from build123d import *

# Parameters (mm, degrees)
CROQUIS1_R              = 12.5
CROQUIS1_R_2            = 0.75
SALIENTE_EXTRUIR1_DEPTH = 10
CROQUIS2_R              = 7.875
SALIENTE_EXTRUIR2_DEPTH = 13
SALIENTE_EXTRUIR3_DEPTH = 8
CROQUIS4_R              = 2
CORTAR_EXTRUIR1_DEPTH   = 32
REDONDEO1_R             = 1


with BuildPart() as part:
    # Croquis1 → Saliente-Extruir1 (new body)
    with BuildSketch(Plane(origin=(0, 0, 0), x_dir=(1, 0, 0), z_dir=(0, 1, 0))):
        Circle(CROQUIS1_R)
        with Locations((7, 0)):
            Circle(CROQUIS1_R_2, mode=Mode.SUBTRACT)
        with Locations((0, -7)):
            Circle(CROQUIS1_R_2, mode=Mode.SUBTRACT)
        with Locations((-7, 0)):
            Circle(CROQUIS1_R_2, mode=Mode.SUBTRACT)
        with Locations((0, 7)):
            Circle(CROQUIS1_R_2, mode=Mode.SUBTRACT)
    extrude(amount=SALIENTE_EXTRUIR1_DEPTH)

    # Croquis2 → Saliente-Extruir2 (add)
    with BuildSketch(Plane(origin=(0, 10, 0), x_dir=(1, 0, 0), z_dir=(0, 1, 0))):
        Circle(CROQUIS2_R)
    extrude(amount=SALIENTE_EXTRUIR2_DEPTH)

    # Croquis3 → Saliente-Extruir3 (add)
    with BuildSketch(Plane(origin=(0, 23, 0), x_dir=(1, 0, 0), z_dir=(0, 1, 0))):
        Polygon((7.5, 0), (3.75, 6.495190528), (-3.75, 6.495190528), (-7.5, 0), (-3.75, -6.495190528), (3.75, -6.495190528), align=None)
    extrude(amount=SALIENTE_EXTRUIR3_DEPTH)

    # Croquis4 → Cortar-Extruir1 (cut, through all)
    with BuildSketch(Plane(origin=(0, 31, 0), x_dir=(1, 0, 0), z_dir=(0, 1, 0))):
        Circle(CROQUIS4_R)
    extrude(amount=-CORTAR_EXTRUIR1_DEPTH, mode=Mode.SUBTRACT)

    # Redondeo1
    redondeo1_edges = [part.edges().sort_by_distance(p)[0] for p in [
        (5.625, 31, 3.247595264),
        (5.625, 31, -3.247595264),
        (0, 31, -6.495190528),
        (-5.625, 31, -3.247595264),
        (-5.625, 31, 3.247595264),
        (0, 31, 6.495190528),
        (-2, 31, 0),
    ]]
    fillet(redondeo1_edges, radius=REDONDEO1_R)


solid = part.part
CAD build for the part. Positions are in the model's coordinates, mm. A direction names the side the tool comes from. Round coordinates to 2 decimals unless told otherwise and drop trailing zeros. Loops run counter-clockwise (first coordinate to the right, second up) from the corner with the lowest first, then second, coordinate; pieces in that order, holes last.
(1) Cut at D-D (z = -7). Give the cut face in (x, y).
(2) Wall check: line 1 along X through (y, z) = (3, 0); line 2 along X through (y, z) = (15, 0) (3 decimals). Give the ranges that are in metal, low to high.
(3) Two-plate mould, pull along Z, no slides. Class faces 5 (the flat face through (0, 26, -6.495)), 6 (the flat face through (-6, 23, 3)), 7 (the flat face through (0, 10, 7)), 8 (the flat face through (0, 26, 6.495)): +Z half, -Z half, draft (parallel to the pull), parting line (faces both ways), or undercut.
(4) Cut at C-C (y = 16). Give the cut face in (x, z) (3 decimals), plus the area to 3 significant figures.
(5) Cut at B-B (y = 6.5). Give the cut face in (x, z).
(6) Cut at A-A (x = 0). Give the cut face in (y, z) (3 decimals), plus the area to 3 significant figures.
(7) Drop flat-ended pins along their axis: pin 1 (3.5 mm diameter, centred on x = 0, y = 28, fed in from +Z); pin 2 (3 mm diameter, centred on x = 6, z = -4.5, fed in from +Y); pin 3 (5 mm diameter, centred on y = 24.5, z = 5.5, fed in from +X); pin 4 (3.5 mm diameter, centred on x = 0, z = 0, fed in from -Y). Give the stop position or say it passes through.
(8) Which spindle directions (+Z, -Z, +X, -X, +Y, -Y) get a long thin tool onto all of the face, cutting with end or side? Do faces 1 (the cylindrical face through (-0.05, 30.7, -6.21)), 2 (the flat face through (5.6, 26.45, 3.29)), 3 (the flat face through (-5.651, 26.451, 3.202)), 4 (the cylindrical face through (-0.163, 4.93, 7.732)). Say none if no direction does.
Findings below:
1. outline: (-10.36, 0) - (-0.75, 0) - (-0.75, 10) - (0.75, 10) - (0.75, 0) - (10.36, 0) - (10.36, 10) - (3.61, 10) - (3.61, 23) - (-3.61, 23) - (-3.61, 10) - (-10.36, 10) - close
2. line 1: x = -12.5 to -7.75, -6.25 to -2, 2 to 6.25, 7.75 to 12.5
2. line 2: x = -7.875 to -2, 2 to 7.875
3. face 5: -Z half
3. face 6: draft
3. face 7: undercut
3. face 8: +Z half
4. outline: circle Ø15.75 at (0, 0); hole circle Ø4 at (0, 0)
4. area: 182 mm2
5. outline: circle Ø25 at (0, 0); hole circle Ø1.5 at (-7, 0); hole circle Ø4 at (0, 0); hole circle Ø1.5 at (0, -7); hole circle Ø1.5 at (0, 7); hole circle Ø1.5 at (7, 0)
6. outline: (0, -12.5) - (10, -12.5) - (10, -7.875) - (23, -7.875) - (23, -6.495) - (30, -6.495) arc R1 ccw to (31, -5.495) - (31, -3) arc R1 ccw to (30, -2) - (0, -2) - (0, -6.25) - (10, -6.25) - (10, -7.75) - (0, -7.75) - close; (0, 2) - (30, 2) arc R1 ccw to (31, 3) - (31, 5.495) arc R1 ccw to (30, 6.495) - (23, 6.495) - (23, 7.875) - (10, 7.875) - (10, 12.5) - (0, 12.5) - (0, 7.75) - (10, 7.75) - (10, 6.25) - (0, 6.25) - close
6. area: 404 mm2
7. pin 1: stops at z = 6.5
7. pin 2: stops at y = 30.89
7. pin 3: stops at x = 7.05
7. pin 4: passes through
8. face 1: -Z, +X, -X, +Y
8. face 2: +Z, +X, +Y
8. face 3: +Z, -X, +Y
8. face 4: -Y
